Can you work these out from the model? Positions are in its coordinate system, mm. Face numbers are marked on the shaded views. A direction names the side the tool comes from. Round coordinates to 2 decimals unless told otherwise and drop trailing zeros. Write each loop counter-clockwise with the first axis right and the second up, starting at its lowest first coordinate (ties: lowest second). Pieces come first, ordered by that corner, then holes. Notation, with made-up numbers: (-16, -25) -> (7, -25) arc R28 ccw to (7, -2) -> close; hole circle Ø9 at (77.5, 52.5). An arc over 180 degrees is marked (long way). Write item = value, one per line. Start each with the question number.
1) If I drill on line 1 (X direction, y = -1.75, z = 5.75); line 2 (X direction, y = 1.25, z = 1); line 3 (Y direction, x = -17.75, z = 1), over which ranges is the centre line in solid material (lowest first)?
2) Imagine slicing it at C-C, the plane x = 2.5. Please give me the cut outline in (y, z), then the cut area to 3 significant figures.
3) Thinking about a two-plate mould opening in Y: for the marked faces 1, 2 and 3, which applies, +Y half, -Y half, draft (parallel to the pull), parting line (faces both ways), or undercut?
4) I'm going to push flat-ended pins straight in: pin 1 (2.5 mm diameter, centred on x = -18.5, z = 6.5, fed in from -Y); pin 2 (0.5 mm diameter, centred on y = -3.5, z = 6, fed in from -X); pin 3 (0.8 mm diameter, centred on y = -4, z = 6.5, fed in from -X); pin 4 (0.8 mm diameter, centred on y = 4, z = 6, fed in from -X). Where does each tip first touch, or does it pass through?
5) Imagine slicing it at B-B, the plane z = 1.75. State how many separate pieces and enclosed holes the cut face has, then the cut area to 3 significant figures.
6) For the marked faces 4, 5, 6 and 7, which set-ups out of +Z, -Z, +X, -X, +Y, -Y let a thin tool reach every point of the face, with its end or its side?
7) Imagine slicing it at D-D, the plane x = -19. Please give me the cut outline in (y, z), then the cut area to 3 significant figures.
8) Imagine slicing it at A-A, the plane x = -25.75. Please give me the cut outline in (y, z).
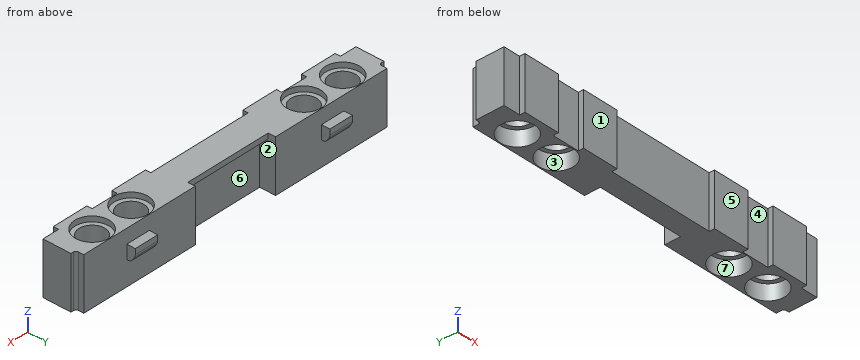
from build123d import *

# Parameters (mm, degrees)
SKETCH1_W           = 64.3
SKETCH1_H           = 6.8
SKETCH1_R           = 2.45
BOSS_EXTRUDE2_DEPTH = 9.9
SKETCH2_R           = 3.25
CUT_EXTRUDE1_DEPTH  = 2.9
CUT_EXTRUDE2_DEPTH  = 11
SKETCH7_W           = 6.9
SKETCH7_H           = 1
BOSS_EXTRUDE3_DEPTH = 9.9
SKETCH8_W           = 16.5
SKETCH8_H           = 6
CUT_EXTRUDE3_DEPTH  = 12
SKETCH9_W           = 16.5
SKETCH9_H           = 1.6
BOSS_EXTRUDE4_DEPTH = 1
SKETCH10_W          = 4.6
SKETCH10_H          = 2.6
BOSS_EXTRUDE5_DEPTH = 1.6
CUT_EXTRUDE4_REACH  = 57.568
FILLET1_R           = 1
CUT_EXTRUDE6_START  = -1
SKETCH13_R          = 3.25
CUT_EXTRUDE6_DEPTH  = 1


with BuildPart() as part:
    # Sketch1 → Boss-Extrude2 (new body)
    with BuildSketch(Plane.XY):
        Rectangle(SKETCH1_W, SKETCH1_H)
        with Locations(Location((-17.75, 0, 0), (0, 0, 180))):
            Circle(SKETCH1_R, mode=Mode.SUBTRACT)
        with Locations(Location((-25.75, 0, 0), (0, 0, 180))):
            Circle(SKETCH1_R, mode=Mode.SUBTRACT)
        with Locations(Location((17.75, 0, 0), (0, 0, 180))):
            Circle(SKETCH1_R, mode=Mode.SUBTRACT)
        with Locations(Location((25.75, 0, 0), (0, 0, 180))):
            Circle(SKETCH1_R, mode=Mode.SUBTRACT)
    extrude(amount=BOSS_EXTRUDE2_DEPTH)

    # Sketch2 → Cut-Extrude1 (cut)
    with BuildSketch(Plane(origin=(0, 0, 0), x_dir=(-1, 0, 0), z_dir=(0, 0, -1))):
        with Locations((-25.75, 0)):
            Circle(SKETCH2_R)
        with Locations((-17.75, 0)):
            Circle(SKETCH2_R)
        with Locations(Location((17.75, 0, 0), (0, 0, 180))):
            Circle(SKETCH2_R)
        with Locations(Location((25.75, 0, 0), (0, 0, 180))):
            Circle(SKETCH2_R)
    extrude(amount=-CUT_EXTRUDE1_DEPTH, mode=Mode.SUBTRACT)

    # Sketch5 → Cut-Extrude2 (cut)
    with BuildSketch(Plane.XY.offset(9.9)):
        with BuildLine():
            Line((32.15, 3.4), (31.15, 3.4))
            Line((31.15, 3.4), (31.15, 2.4))
            ThreePointArc((31.15, 2.4), (31.296446609, 2.046446609), (31.65, 1.9))
            Line((31.65, 1.9), (32.15, 1.9))
            Line((32.15, 1.9), (32.15, 3.4))
        make_face()
        with BuildLine():
            Line((-32.15, 3.4), (-32.15, 1.9))
            Line((-32.15, 1.9), (-31.65, 1.9))
            ThreePointArc((-31.65, 1.9), (-31.296446609, 2.046446609), (-31.15, 2.4))
            Line((-31.15, 2.4), (-31.15, 3.4))
            Line((-31.15, 3.4), (-32.15, 3.4))
        make_face()
    extrude(amount=-CUT_EXTRUDE2_DEPTH, mode=Mode.SUBTRACT)

    # Sketch7 → Boss-Extrude3 (add)
    with BuildSketch(Plane.XY.offset(9.9)):
        with Locations((-25.5, -3.9)):
            Rectangle(SKETCH7_W, SKETCH7_H)
        with Locations((-13.45, -3.9)):
            Rectangle(SKETCH7_W, SKETCH7_H)
        with Locations((13.45, -3.9)):
            Rectangle(SKETCH7_W, SKETCH7_H)
        with Locations((25.5, -3.9)):
            Rectangle(SKETCH7_W, SKETCH7_H)
    extrude(amount=-BOSS_EXTRUDE3_DEPTH)

    # Sketch8 → Cut-Extrude3 (cut)
    with BuildSketch(Plane.XY.offset(9.9)):
        with Locations((0, 3.4)):
            Rectangle(SKETCH8_W, SKETCH8_H)
    extrude(amount=-CUT_EXTRUDE3_DEPTH, mode=Mode.SUBTRACT)

    # Sketch9 → Boss-Extrude4 (add)
    with BuildSketch(Plane.XY.offset(9.9)):
        with Locations((0, 1.2)):
            Rectangle(SKETCH9_W, SKETCH9_H)
    extrude(amount=-BOSS_EXTRUDE4_DEPTH)

    # Sketch10 → Boss-Extrude5 (add)
    with BuildSketch(Plane(origin=(0, 3.4, 0), x_dir=(1, 0, 0), z_dir=(0, 1, 0))):
        with Locations((-20, -5.9)):
            Rectangle(SKETCH10_W, SKETCH10_H)
        with Locations((20, -5.9)):
            Rectangle(SKETCH10_W, SKETCH10_H)
    extrude(amount=BOSS_EXTRUDE5_DEPTH)

    # Cut-Extrude4: up to this face of the body (flat: up to its plane)
    cut_extrude4_end = Plane(part.part.faces().sort_by_distance((22.3, 4.2, 5.9))[0])
    # Sketch11 → Cut-Extrude4 (cut, up to the picked face)
    with BuildSketch(Plane.ZY.offset(22.3), mode=Mode.PRIVATE) as cut_extrude4_sk1:
        Polygon((4.6, 4.2), (5.9, 5), (4.6, 5), align=None)
    cut_extrude4_tool1 = split(extrude(cut_extrude4_sk1.sketch, amount=-CUT_EXTRUDE4_REACH, mode=Mode.PRIVATE), bisect_by=cut_extrude4_end, keep=Keep.BOTH, mode=Mode.PRIVATE)
    add(cut_extrude4_tool1.solids().sort_by(Axis((-22.3, 4.733333, 5.033333), (1, 0, 0)))[0], mode=Mode.SUBTRACT)

    # Fillet1
    fillet1_edges = [part.edges().sort_by_distance(p)[0] for p in [
        (-20, 5, 5.9),
        (-20, 4.2, 4.6),
        (20, 5, 5.9),
        (20, 4.2, 4.6),
    ]]
    fillet(fillet1_edges, radius=FILLET1_R)

    # Sketch13 → Cut-Extrude6 (cut)
    with BuildSketch(Plane.XY.offset(9.9).offset(CUT_EXTRUDE6_START)):
        with Locations((-25.75, 0)):
            Circle(SKETCH13_R)
        with Locations((-17.75, 0)):
            Circle(SKETCH13_R)
        with Locations(Location((25.75, 0, 0), (0, 0, 180))):
            Circle(SKETCH13_R)
        with Locations(Location((17.75, 0, 0), (0, 0, 180))):
            Circle(SKETCH13_R)
    extrude(amount=CUT_EXTRUDE6_DEPTH, mode=Mode.SUBTRACT)


solid = part.part
Reported:
q1.line_1 = -32.15 to -27.46, -24.04 to -19.46, -16.04 to 16.04, 19.46 to 24.04, 27.46 to 32.15
q1.line_2 = -32.15 to -28.75, -22.75 to -20.75, -14.75 to -8.25, 8.25 to 14.75, 20.75 to 22.75, 28.75 to 32.15
q1.line_3 = -3.4 to -3.25, 3.25 to 3.4
q2.outline = (-3.4, 0) -> (0.4, 0) -> (0.4, 8.9) -> (2, 8.9) -> (2, 9.9) -> (-3.4, 9.9) -> close
q2.area = 39.2 mm²
q3.face_1 = -Y half
q3.face_2 = draft
q3.face_3 = undercut
q4.pin_1 = -3.4
q4.pin_2 = -32.15
q4.pin_3 = -28.95
q4.pin_4 = -22.3
q5.separate_pieces = 1
q5.enclosed_holes = 4
q5.area = 280 mm²
q6.face_4 = +Z, -Z, -Y
q6.face_5 = +Z, -Z, +X, -X, -Y
q6.face_6 = -Z, +Y
q6.face_7 = -Z
q7.outline = (-3.4, 0) -> (-3, 0) -> (-3, 2.9) -> (-2.11, 2.9) -> (-2.11, 8.9) -> (-3, 8.9) -> (-3, 9.9) -> (-3.4, 9.9) -> close; (2.11, 2.9) -> (3, 2.9) -> (3, 0) -> (3.4, 0) -> (3.4, 4.6) -> (3.64, 4.6) arc R1 ccw to (4.49, 5.08) -> (4.85, 5.66) arc R1 ccw to (5, 6.18) -> (5, 7.2) -> (3.4, 7.2) -> (3.4, 9.9) -> (3, 9.9) -> (3, 8.9) -> (2.11, 8.9) -> close
q7.area = 22.2 mm²
q8.outline = (-4.4, 0) -> (-3.25, 0) -> (-3.25, 2.9) -> (-2.45, 2.9) -> (-2.45, 8.9) -> (-3.25, 8.9) -> (-3.25, 9.9) -> (-4.4, 9.9) -> close; (2.45, 2.9) -> (3.25, 2.9) -> (3.25, 0) -> (3.4, 0) -> (3.4, 9.9) -> (3.25, 9.9) -> (3.25, 8.9) -> (2.45, 8.9) -> close
